Autodesk Inventor part; units mm, degrees
ref_plane "YZ Plane" through (0, 0, 0) normal (1, 0, 0) x (0, 1, 0)
ref_plane "XZ Plane" through (0, 0, 0) normal (0, 1, 0) x (-1, 0, 0)
ref_plane "XY Plane" through (0, 0, 0) normal (0, 0, 1) x (1, 0, 0)
sketch "Sketch2" plane through (0, 0, 0) normal (1, 0, 0) x (0, 1, 0)
  line L0 (0, 0) -> (44.2, 0)
  line L1 (44.2, 0) -> (44.2, -2)
  line L2 (44.2, -2) -> (2, -15)
  line L3 (2, -15) -> (0, -15)
  line L4 (0, -15) -> (0, 0)
  dimension "d0" = 44.2
  dimension "d1" = 2
  dimension "d2" = 2
  dimension "d3" = 15
extrude "Extrusion1" add sketch "Sketch2" along normal blind 20
sketch "Sketch3" plane through (0, 0, -15) normal (0, -1, 0) x (1, 0, 0)
  line L0 (0, 15) -> (20, 15)
  line L1 (0, 15) -> (20, 0) construction
  line L2 (0, 0) -> (0, 13)
  line L3 (20, 15) -> (0, 0) construction
  circle A0 centre (10, 7.5) radius 2
  dimension "d6" = 4
extrude "Extrusion2" cut sketch "Sketch3" against normal through all
sketch "Sketch4" plane through (0, 0, 0) normal (0, 0, 1) x (1, 0, 0)
  line L0 (20, 2) -> (20, 44.2)
  line L1 (20, 44.2) -> (0, 0) construction
  line L2 (20, 0) -> (20, 2)
  line L3 (0, 2) -> (0, 44.2)
  line L4 (20, 0) -> (0, 44.2) construction
  circle A0 centre (10, 22.1) radius 2
  dimension "d9" = 4
extrude "Extrusion3" cut sketch "Sketch4" against normal through all
properties part number "MM3_vertical"
Can you work these out from the model? Positions are in its coordinate system, mm. A direction names the side the tool comes from. Give positions to 0.01 mm unless a question says otherwise; leave off trailing zeros. Write each loop counter-clockwise with the first axis right and the second up, starting at its lowest first coordinate (ties: lowest second). Pieces come first, ordered by that corner, then holes. Notation, with made-up numbers: (-12.5, 36) - (45.5, 36) arc R19 ccw to (45.5, 53) - close; hole circle Ø11 at (20, 32). An arc over 180 degrees is marked (long way). Write item = value, one per line. Start each with the question number.
1. Imagine slicing it at B-B (x = 16.5). Please give me the cut outline in (y, z), and give its area (3 significant figures).
2. Imagine slicing it at C-C (z = -2.5). Please give me the cut outline in (x, y).
3. For pin 1 (4.5 mm diameter, centred on x = 10, z = -7.5, fed in from -Y); pin 2 (1 mm diameter, centred on x = 14.5, y = 30, fed in from -Z); pin 3 (1 mm diameter, centred on x = 4.5, y = 12.5, fed in from -Z); pin 4 (6 mm diameter, centred on x = 7.5, y = 26, fed in from -Z), each with a flat end and sliding along its axis, tell me the tip position at first contact or that it passes through.
4. Please list where these lines run through material, in increasing order: line 1 (X direction, y = 25.75, z = -7.5); line 2 (Y direction, x = 10, z = -1.75); line 3 (X direction, y = 13.5, z = -7).
5. On a 3-axis mill with a long thin cutter (end or side, diameter ignored), from which of +Z, -Z, +X, -X, +Y, -Y can I reach the whole of each face in a straight line? I mean faces 1 (the face through (11.973, 21.77, -8.511)), 2 (the face through (7.638, 23.395, -8.409)). Say none if no direction works.
6. Imagine slicing it at D-D (y = 10). Please give me the cut outline in (x, z).
7. Thinking about a two-plate mould opening in X: for faces 3 (the face through (7.6, 21.8, 0)), 4 (the face through (8.4, 20.9, -2.9)), 5 (the face through (20, 17, -6)), which applies, released by +X, released by -X, zero draft, split by the parting line, or undercut?
8. Imagine slicing it at A-A (x = 10). Please give me the cut outline in (y, z).
Worked answers:
q1.outline = (0, -15) - (2, -15) - (44.2, -2) - (44.2, 0) - (0, 0) - close
q1.area = 389 mm2
q2.outline = (0, 0) - (20, 0) - (20, 42.58) - (0, 42.58) - close; hole circle Ø4 at (10, 22.1)
q3.pin_1 = 0
q3.pin_2 = -6.53
q3.pin_3 = -11.92
q3.pin_4 = -8.53
q4.line_1 = 0 to 8, 12 to 20
q4.line_2 = 0 to 20.1, 24.1 to 44.2
q4.line_3 = 0 to 8.06, 11.94 to 20
q5.face_1 = +Z, -Z
q5.face_2 = -Z, +X, -X, +Y
q6.outline = (0, -12.54) - (20, -12.54) - (20, 0) - (0, 0) - close; hole circle Ø4 at (10, -7.5)
q7.face_3 = zero draft
q7.face_4 = undercut
q7.face_5 = released by +X
q8.outline = (0, -15) - (2, -15) - (19.85, -9.5) - (0, -9.5) - close; (0, -5.5) - (20.1, -5.5) - (20.1, 0) - (0, 0) - close; (24.1, -5.5) - (32.84, -5.5) - (44.2, -2) - (44.2, 0) - (24.1, 0) - close
